```python
from build123d import *

# Parameters (mm, degrees)
SKETCH1_W                = 7
SKETCH1_H                = 5
BOSS_EXTRUDE1_DEPTH      = 5
HOLE1_D                  = 1.05
HOLE1_CBORE_D            = 1.3
HOLE1_CBORE_DEPTH        = 1.2
SKETCH20_W               = 5
SKETCH20_H               = 2.5
CUT_EXTRUDE11_DEPTH      = 2
M1_0X0_25_TAPPED_HOLE1_D = 0.75
SKETCH37_W               = 5
SKETCH37_H               = 2.5
CUT_EXTRUDE13_DEPTH      = 2
CUT_EXTRUDE15_DEPTH      = 3
CUT_EXTRUDE16_DEPTH      = 9.124038405
SKETCH45_R               = 0.375
CUT_EXTRUDE18_DEPTH      = 0.5
SKETCH44_W               = 0.852349788
SKETCH44_H               = 0.8
CUT_EXTRUDE19_DEPTH      = 4.5


with BuildPart() as part:
    # Sketch1 → Boss-Extrude1 (new body)
    with BuildSketch(Plane(origin=(0, 4, 0), x_dir=(-1, 0, 0), z_dir=(0, 1, 0))):
        with Locations((-3.5, 2.5)):
            Rectangle(SKETCH1_W, SKETCH1_H)
    extrude(amount=-BOSS_EXTRUDE1_DEPTH)

    # Hole1 (through all)
    with Locations(Plane(origin=(0, 0, 0), x_dir=(-1, 0, 0), z_dir=(0, 0, -1))):
        with Locations((-5.7, 0.5), (-0.7, 0.5)):
            CounterBoreHole(HOLE1_D / 2, HOLE1_CBORE_D / 2, HOLE1_CBORE_DEPTH)

    # Sketch20 → Cut-Extrude11 (cut)
    with BuildSketch(Plane(origin=(7, 0, 0), x_dir=(0, 0, -1), z_dir=(1, 0, 0))):
        with Locations((-2.5, 2.75)):
            Rectangle(SKETCH20_W, SKETCH20_H)
    extrude(amount=-CUT_EXTRUDE11_DEPTH, mode=Mode.SUBTRACT)

    # M1.0x0.25 Tapped Hole1 (through all)
    with Locations(Plane(origin=(0, 0, 0), x_dir=(-1, 0, 0), z_dir=(0, 0, -1))):
        with Locations((-3.2, 0.5)):
            Hole(M1_0X0_25_TAPPED_HOLE1_D / 2)

    # Sketch37 → Cut-Extrude13 (cut)
    with BuildSketch(Plane.ZY):
        with Locations((2.5, 2.752068207)):
            Rectangle(SKETCH37_W, SKETCH37_H)
    extrude(amount=-CUT_EXTRUDE13_DEPTH, mode=Mode.SUBTRACT)

    # Sketch41 → Cut-Extrude15 (cut)
    with BuildSketch(Plane(origin=(0, 4, 0), x_dir=(1, 0, 0), z_dir=(0, 1, 0))):
        Polygon((5, -2.6), (3.822078101, -2.05), (3.822078101, -4.55), (5, -4), align=None)
    extrude(amount=-CUT_EXTRUDE15_DEPTH, mode=Mode.SUBTRACT)

    # Sketch43 → Cut-Extrude16 (cut, through all)
    with BuildSketch(Plane.ZY.offset(-2)):
        Polygon((0, 2.302068207), (0.606217783, 1.952068207), (0.606217783, 3.452068207), (0, 3.102068207), align=None)
    extrude(amount=-CUT_EXTRUDE16_DEPTH, mode=Mode.SUBTRACT)

    # Sketch45 → Cut-Extrude18 (cut)
    with BuildSketch(Plane(origin=(0, 1, 0), x_dir=(1, 0, 0), z_dir=(0, 1, 0))):
        with Locations(Location((4.404643106, -3.280769975, 0), (0, 0, 270))):
            Circle(SKETCH45_R)
    extrude(amount=-CUT_EXTRUDE18_DEPTH, mode=Mode.SUBTRACT)

    # Sketch44 → Cut-Extrude19 (cut)
    with BuildSketch(Plane(origin=(0, 0, 0.606217783), x_dir=(-1, 0, 0), z_dir=(0, 0, -1))):
        with Locations((-2.426174894, 2.616682439)):
            Rectangle(SKETCH44_W, SKETCH44_H)
    extrude(amount=-CUT_EXTRUDE19_DEPTH, mode=Mode.SUBTRACT)


solid = part.part
```
The listing builds one solid part. Answer for the finished solid, in the listing's coordinates (mm). A direction names the side the tool comes from. Coordinates: 2 decimals unless noted, no trailing zeros. Loops run counter-clockwise (first coordinate to the right, second up) from the corner with the lowest first, then second, coordinate; pieces in that order, holes last. Notation, with made-up numbers: M 75.5,18 L 79.5,18 A11 ccw 79.5,34 Z; hole C -21,47.25 d11. An arc over 180 degrees is marked long. Answer as CSV lines item,"result". Start each with the question number.
(1) Find the intervals of material crossed by L1, parallel to Y at x = 3.2, z = 2.9 (3 decimals); L2, parallel to Y at x = 5.7, z = 3.9 (3 decimals); L3, parallel to X at y = 2.7, z = 1.65, in increasing order. Write a range as [from, to].
(2) The part is cut by section B-B (z = 0.9). Give the vertices of the cut face in (x, y) (3 decimals).
(3) The part is cut by section D-D (x = 0.7). Give the vertices of the cut face in (y, z) (3 decimals).
(4) The part is cut by section C-C (y = 2.4). Give the vertices of the cut face in (x, z).
(5) For faces 4 (the flat face through (2.4, 3.017, 2.8)), 5 (the cylindrical face through (5.1, 0.25, 0.59)), 6 (the flat face through (5, 2.8, 4.5)), 7 (the flat face through (4.4, 2.52, 4.28)), determine the directions among +Z, -Z, +X, -X, +Y, -Y from which every point of the face is accessible in a straight line to the end or side of a thin tool.
(6) The mould has two halves that part along Y. Classify faces 1 (the cylindrical face through (0.942, 0.034, 3.127)), 2 (the flat face through (3, 4, 3)), 3 (the flat face through (4, 0, 0)): pulls with the +Y half, pulls with the -Y half, needs draft (parallel to the pull), parting line crosses it, or undercut.
(7) Given pin 1 (0.8 mm diameter, centred on x = 0.7, y = 0.5, fed in from +Z), flat-ended and moving along its own axis, determine where the tip first touches the part or whether it passes through.
(8) The part is cut by section A-A (x = 5.7). Give the vertices of the cut face in (y, z) (3 decimals), and give its area (3 significant figures).
Determined:
1,L1,"[-1, 0.125], [0.875, 4]"
1,L2,"[-1, -0.025], [1.025, 1.5]"
1,L3,"[2.85, 5]"
2,outline,"M 0,-1 L 7,-1 L 7,1.5 L 5,1.5 L 5,4 L 2,4 L 2,3.017 L 2.852,3.017 L 2.852,2.217 L 2,2.217 L 2,1.502 L 0,1.502 Z; hole C 0.7,0.5 d1.3; hole C 3.2,0.5 d0.75; hole C 5.7,0.5 d1.3"
3,outline,"M -1,0 L -0.15,0 L -0.15,1.2 L -0.025,1.2 L -0.025,5 L -1,5 Z; M 1.025,1.2 L 1.15,1.2 L 1.15,0 L 1.502,0 L 1.502,5 L 1.025,5 Z"
4,outline,"M 2.85,0.61 L 5,0.61 L 5,2.6 L 3.82,2.05 L 3.82,4.55 L 5,4 L 5,5 L 2.85,5 Z"
5,face 4,"+Z, -Z, -X"
5,face 5,"-Z"
5,face 6,"+Z, -Z, +X, +Y"
5,face 7,"+Y"
6,face 1,"undercut"
6,face 2,"pulls with the +Y half"
6,face 3,"needs draft"
7,pin 1,"through"
8,outline,"M -1,0 L -0.15,0 L -0.15,1.2 L -0.025,1.2 L -0.025,5 L -1,5 Z; M 1.025,1.2 L 1.15,1.2 L 1.15,0 L 1.5,0 L 1.5,5 L 1.025,5 Z"
8,area,"6.95 mm2"
